```python
from build123d import *

# Parameters (mm, degrees)
SKETCH1_R           = 40
SKETCH1_R_2         = 1.75
SKETCH1_R_3         = 23
BOSS_EXTRUDE1_DEPTH = 3.5


with BuildPart() as part:
    # Sketch1 → Boss-Extrude1 (new body)
    with BuildSketch(Plane(origin=(0, 0, 0), x_dir=(1, 0, 0), z_dir=(0, 1, 0))):
        Circle(SKETCH1_R)
        with Locations((10, 35)):
            Circle(SKETCH1_R_2, mode=Mode.SUBTRACT)
        with Locations((-10, 35)):
            Circle(SKETCH1_R_2, mode=Mode.SUBTRACT)
        with Locations((10, -35)):
            Circle(SKETCH1_R_2, mode=Mode.SUBTRACT)
        with Locations((-10, -35)):
            Circle(SKETCH1_R_2, mode=Mode.SUBTRACT)
        Circle(SKETCH1_R_3, mode=Mode.SUBTRACT)
    extrude(amount=BOSS_EXTRUDE1_DEPTH)


solid = part.part
```
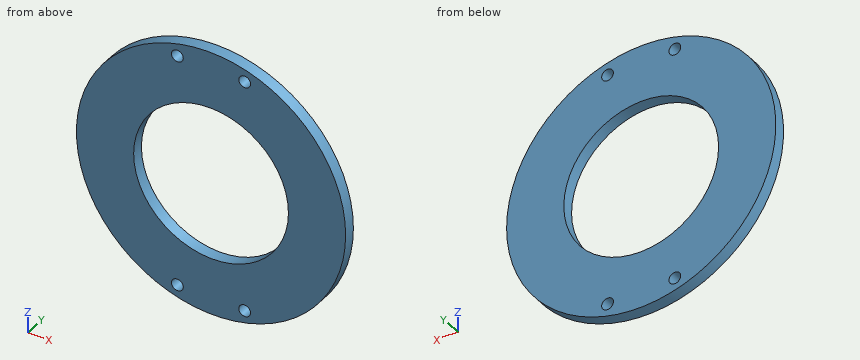
The listing builds one solid part. Answer for the finished solid, in the listing's coordinates (mm). Give positions to 0.01 mm unless a question says otherwise; leave off trailing zeros. Order: outer loops, then holes, each group sorted by start corner. A loop starts at its lowest first (then second) coordinate and runs counter-clockwise, first axis right, second up.
1) Consider line 1 along Z through (x, y) = (-10, 1.7); line 2 along X through (y, z) = (0.95, 0); line 3 along X through (y, z) = (1, 35). Determine where each line is inside the solid, lowest interval first.
Reported:
line 1: z = -38.73 to -36.75, -33.25 to -20.71, 20.71 to 33.25, 36.75 to 38.73
line 2: x = -40 to -23, 23 to 40
line 3: x = -19.36 to -11.75, -8.25 to 8.25, 11.75 to 19.36
2) Find section A-A on z = 0. Write down the section's boundary in (x, y).
Reported:
outline: (-40, 0) - (-23, 0) - (-23, 3.5) - (-40, 3.5) - close; (23, 0) - (40, 0) - (40, 3.5) - (23, 3.5) - close
3) Find section C-C on z = 35. Write down the section's boundary in (x, y), then the cut area to 3 significant figures.
Reported:
outline: (-19.36, 0) - (-11.75, 0) - (-11.75, 3.5) - (-19.36, 3.5) - close; (-8.25, 0) - (8.25, 0) - (8.25, 3.5) - (-8.25, 3.5) - close; (11.75, 0) - (19.36, 0) - (19.36, 3.5) - (11.75, 3.5) - close
area: 111 mm2
4) Given P1, Ø3, axis at x = 10, z = -35, coming from the -Y side; P2, Ø1, axis at x = -9, y = 1, coming from the -Z side, each flat-ended and moving along its own axis, determine where each tip first touches the part or whether it passes through.
Reported:
P1: passes through
P2: stops at z = -39.09
5) Find section D-D on z = -24. Write down the section's boundary in (x, y), then the cut area to 3 significant figures.
Reported:
outline: (-32, 0) - (32, 0) - (32, 3.5) - (-32, 3.5) - close
area: 224 mm2
6) Find section B-B on x = 3. Write down the section's boundary in (y, z).
Reported:
outline: (0, -39.89) - (3.5, -39.89) - (3.5, -22.8) - (0, -22.8) - close; (0, 22.8) - (3.5, 22.8) - (3.5, 39.89) - (0, 39.89) - close
